Part model, mm, in its own coordinate system. Coordinates: 2 decimals unless noted, no trailing zeros.
from build123d import *

# Parameters (mm, degrees)
SKETCH1_W           = 430
SKETCH1_H           = 500
BOSS_EXTRUDE1_DEPTH = 1.5
SKETCH12_R          = 1.95
CUT_EXTRUDE3_DEPTH  = 50.8
SKETCH6_R           = 1.95
CUT_EXTRUDE4_DEPTH  = 50.8
SKETCH7_R           = 1.95
CUT_EXTRUDE5_DEPTH  = 50.8
FILLET1_R           = 2
CUT_EXTRUDE6_DEPTH  = 10


with BuildPart() as part:
    # Sketch1 → Boss-Extrude1 (new body)
    with BuildSketch(Plane(origin=(0, 0, 0), x_dir=(1, 0, 0), z_dir=(0, 1, 0))):
        Rectangle(SKETCH1_W, SKETCH1_H)
    extrude(amount=BOSS_EXTRUDE1_DEPTH)

    # Sketch12 → Cut-Extrude3 (cut)
    with BuildSketch(Plane(origin=(0, 0, 0), x_dir=(-1, 0, 0), z_dir=(0, -1, 0))):
        with Locations((-185, -175)):
            Circle(SKETCH12_R)
        with Locations((-205, 170)):
            Circle(SKETCH12_R)
        with Locations((-205, -175)):
            Circle(SKETCH12_R)
        with Locations((-185, 170)):
            Circle(SKETCH12_R)
        with Locations((205, -175)):
            Circle(SKETCH12_R)
        with Locations((185, 175)):
            Circle(SKETCH12_R)
        with Locations((205, 175)):
            Circle(SKETCH12_R)
        with Locations((185, -175)):
            Circle(SKETCH12_R)
    extrude(amount=-CUT_EXTRUDE3_DEPTH, mode=Mode.SUBTRACT)

    # Sketch6 → Cut-Extrude4 (cut)
    with BuildSketch(Plane(origin=(0, 1.5, 0), x_dir=(1, 0, 0), z_dir=(0, 1, 0))):
        with Locations((92.292697989, -28)):
            Circle(SKETCH6_R)
        with Locations((42.292697989, -28)):
            Circle(SKETCH6_R)
        with Locations((92.292697989, -178)):
            Circle(SKETCH6_R)
        with Locations((42.292697989, -178)):
            Circle(SKETCH6_R)
    extrude(amount=-CUT_EXTRUDE4_DEPTH, mode=Mode.SUBTRACT)

    # Sketch7 → Cut-Extrude5 (cut)
    with BuildSketch(Plane(origin=(0, 1.5, 0), x_dir=(1, 0, 0), z_dir=(0, 1, 0))):
        with Locations((-114.979961576, 95.192396061)):
            Circle(SKETCH7_R)
        with Locations((-54.979961576, 95.192396061)):
            Circle(SKETCH7_R)
        with Locations((-54.979961576, 0.192396061)):
            Circle(SKETCH7_R)
        with Locations((-114.979961576, 0.192396061)):
            Circle(SKETCH7_R)
    extrude(amount=-CUT_EXTRUDE5_DEPTH, mode=Mode.SUBTRACT)

    # Fillet1
    fillet1_edges = [part.edges().sort_by_distance(p)[0] for p in [
        (215, 0.75, 250),
        (-215, 0.75, 250),
        (-215, 0.75, -250),
        (215, 0.75, -250),
    ]]
    fillet(fillet1_edges, radius=FILLET1_R)

    # Sketch13 → Cut-Extrude6 (cut)
    with BuildSketch(Plane.XZ):
        with BuildLine():
            ThreePointArc((128.328231895, 194.409545443), (128.328231895, 201.480613255), (121.257164083, 201.480613255))
            Line((121.257164083, 201.480613255), (6.257164083, 86.480613255))
            ThreePointArc((6.257164083, 86.480613255), (6.257164083, 79.409545443), (13.328231895, 79.409545443))
            Line((13.328231895, 79.409545443), (128.328231895, 194.409545443))
        make_face()
        with BuildLine():
            ThreePointArc((114.891555161, 206.259007204), (114.891555161, 214.740992796), (106.409569569, 214.740992796))
            Line((106.409569569, 214.740992796), (5.551705193, 113.883128419))
            ThreePointArc((5.551705193, 113.883128419), (5.551705193, 105.401142828), (14.033690785, 105.401142828))
            Line((14.033690785, 105.401142828), (114.891555161, 206.259007204))
        make_face()
        with BuildLine():
            ThreePointArc((128.328231895, 169.409545443), (128.328231895, 176.480613255), (121.257164083, 176.480613255))
            Line((121.257164083, 176.480613255), (6.257164083, 61.480613255))
            ThreePointArc((6.257164083, 61.480613255), (6.257164083, 54.409545443), (13.328231895, 54.409545443))
            Line((13.328231895, 54.409545443), (128.328231895, 169.409545443))
        make_face()
        with BuildLine():
            ThreePointArc((128.328231895, 144.409545443), (128.328231895, 151.480613255), (121.257164083, 151.480613255))
            Line((121.257164083, 151.480613255), (6.257164083, 36.480613255))
            ThreePointArc((6.257164083, 36.480613255), (6.257164083, 29.409545443), (13.328231895, 29.409545443))
            Line((13.328231895, 29.409545443), (128.328231895, 144.409545443))
        make_face()
        with BuildLine():
            ThreePointArc((7.050771569, 137.384062043), (5.156114678, 129.125444121), (13.4147326, 131.020101013))
            Line((13.4147326, 131.020101013), (89.712651072, 207.318019485))
            ThreePointArc((89.712651072, 207.318019485), (89.712651072, 213.681980515), (83.348690041, 213.681980515))
            Line((83.348690041, 213.681980515), (7.050771569, 137.384062043))
        make_face()
        with BuildLine():
            ThreePointArc((128.328231895, 119.409545443), (128.328231895, 126.480613255), (121.257164083, 126.480613255))
            Line((121.257164083, 126.480613255), (6.257164083, 11.480613255))
            ThreePointArc((6.257164083, 11.480613255), (6.257164083, 4.409545443), (13.328231895, 4.409545443))
            Line((13.328231895, 4.409545443), (128.328231895, 119.409545443))
        make_face()
        with BuildLine():
            ThreePointArc((129.178407924, 95.256425689), (129.178407924, 102.327493501), (122.107340112, 102.327493501))
            Line((122.107340112, 102.327493501), (18.815380517, -0.964466094))
            ThreePointArc((18.815380517, -0.964466094), (18.815380517, -8.035533906), (25.886448329, -8.035533906))
            Line((25.886448329, -8.035533906), (129.178407924, 95.256425689))
        make_face()
        with BuildLine():
            ThreePointArc((64.186096271, 206.964466094), (64.186096271, 214.035533906), (57.115028459, 214.035533906))
            Line((57.115028459, 214.035533906), (6.257164083, 163.17766953))
            ThreePointArc((6.257164083, 163.17766953), (6.257164083, 156.106601718), (13.328231895, 156.106601718))
            Line((13.328231895, 156.106601718), (64.186096271, 206.964466094))
        make_face()
        with BuildLine():
            ThreePointArc((128.328231895, 71.106601718), (128.328231895, 78.17766953), (121.257164083, 78.17766953))
            Line((121.257164083, 78.17766953), (42.115028459, -0.964466094))
            ThreePointArc((42.115028459, -0.964466094), (42.115028459, -8.035533906), (49.186096271, -8.035533906))
            Line((49.186096271, -8.035533906), (128.328231895, 71.106601718))
        make_face()
        with BuildLine():
            ThreePointArc((128.434071453, 42.778300689), (128.450410182, 50.077386347), (121.151324524, 50.093725076))
            Line((121.151324524, 50.093725076), (70.101549086, -0.728014801))
            ThreePointArc((70.101549086, -0.728014801), (70.211536159, -8.378376983), (77.854021235, -8.014288369))
            Line((77.854021235, -8.014288369), (80.943634504, -4.5))
            Line((80.943634504, -4.5), (128.434071453, 42.778300689))
        make_face()
        with BuildLine():
            ThreePointArc((39.186096271, 206.964466094), (39.186090231, 214.035539946), (32.11501638, 214.035521827))
            Line((32.11501638, 214.035521827), (28.579518712, 210.5))
            Line((28.579518712, 210.5), (6.257188241, 188.17766953))
            ThreePointArc((6.257188241, 188.17766953), (6.257176162, 181.106613797), (13.328231895, 181.106601718))
            Line((13.328231895, 181.106601718), (39.186096271, 206.964466094))
        make_face()
        with BuildLine():
            ThreePointArc((128.328231895, 21.106601718), (128.328231895, 28.17766953), (121.257164083, 28.17766953))
            Line((121.257164083, 28.17766953), (92.115028459, -0.964466094))
            ThreePointArc((92.115028459, -0.964466094), (92.115028459, -8.035533906), (99.186096271, -8.035533906))
            Line((99.186096271, -8.035533906), (128.328231895, 21.106601718))
        make_face()
        with BuildLine():
            ThreePointArc((128.328449123, -3.893615534), (128.328449135, 3.177669518), (121.257164083, 3.17766953))
            Line((121.257164083, 3.17766953), (117.115028459, -0.964466094))
            ThreePointArc((117.115028459, -0.964466094), (117.11493575, -8.035441194), (124.185910844, -8.035719323))
            Line((124.185910844, -8.035719323), (128.328449123, -3.893615534))
        make_face()
        with BuildLine():
            Line((-60.282225947, -95.192396061), (-54.979961576, -89.89013169))
            Line((-54.979961576, -89.89013169), (-52.328312545, -87.235758493))
            ThreePointArc((-52.328312545, -87.235758493), (-52.33035331, -81.93586188), (-57.630250273, -81.936542135))
            Line((-57.630250273, -81.936542135), (-68.235815502, -92.542107364))
            ThreePointArc((-68.235815502, -92.542107364), (-68.236495757, -97.842004327), (-62.936599144, -97.844045092))
            Line((-62.936599144, -97.844045092), (-60.282225947, -95.192396061))
        make_face()
        with BuildLine():
            Line((-79.432380406, -95.192396061), (-52.328311176, -68.084345475))
            ThreePointArc((-52.328311176, -68.084345475), (-52.332091228, -62.778048343), (-57.638379198, -62.788609103))
            Line((-57.638379198, -62.788609103), (-87.242774375, -92.549084557))
            ThreePointArc((-87.242774375, -92.549084557), (-87.193524879, -97.884311066), (-81.85941362, -97.764626075))
            Line((-81.85941362, -97.764626075), (-79.432380406, -95.192396061))
        make_face()
        with BuildLine():
            Line((-98.589718565, -95.192396061), (-54.979961576, -51.582639071))
            Line((-54.979961576, -51.582639071), (-52.328311176, -48.930599166))
            ThreePointArc((-52.328311176, -48.930599166), (-52.332818712, -43.623576712), (-57.639827781, -43.636319812))
            Line((-57.639827781, -43.636319812), (-106.244222321, -92.550540935))
            ThreePointArc((-106.244222321, -92.550540935), (-106.146641992, -97.928953998), (-100.773557317, -97.670477564))
            Line((-100.773557317, -97.670477564), (-98.589718565, -95.192396061))
        make_face()
        with BuildLine():
            Line((-111.925519092, -89.374450278), (-52.328311147, -29.777242332))
            ThreePointArc((-52.328311147, -29.777242332), (-52.310450744, -24.491922995), (-57.595528665, -24.438342602))
            Line((-57.595528665, -24.438342602), (-117.992839573, -83.224558883))
            ThreePointArc((-117.992839573, -83.224558883), (-118.054977502, -89.353737319), (-111.925519092, -89.374450278))
        make_face()
        with BuildLine():
            Line((-112.328311147, -70.623496023), (-52.374195212, -10.669380088))
            ThreePointArc((-52.374195212, -10.669380088), (-52.374195212, -5.457847361), (-57.58572794, -5.457847361))
            Line((-57.58572794, -5.457847361), (-114.979961576, -62.668544735))
            Line((-114.979961576, -62.668544735), (-117.631612006, -65.320195164))
            ThreePointArc((-117.631612006, -65.320195164), (-117.631612006, -70.623496023), (-112.328311147, -70.623496023))
        make_face()
        with BuildLine():
            Line((-112.328311147, -51.123496023), (-63.949411742, -2.744596618))
            ThreePointArc((-63.949411742, -2.744596618), (-63.936748679, 2.34707829), (-69.028297614, 2.385067165))
            Line((-69.028297614, 2.385067165), (-71.657559216, -0.192396061))
            Line((-71.657559216, -0.192396061), (-114.979961576, -43.514798421))
            Line((-114.979961576, -43.514798421), (-117.432443337, -45.634975273))
            ThreePointArc((-117.432443337, -45.634975273), (-117.726028226, -51.025591461), (-112.328311147, -51.123496023))
        make_face()
        with BuildLine():
            Line((-112.328311147, -31.623496023), (-83.202607923, -2.497792799))
            ThreePointArc((-83.202607923, -2.497792799), (-83.175365618, 2.085432584), (-87.75794332, 2.167155652))
            Line((-87.75794332, 2.167155652), (-117.567824527, -26.25790651))
            ThreePointArc((-117.567824527, -26.25790651), (-117.662945906, -31.591787403), (-112.328311147, -31.623496023))
        make_face()
        with BuildLine():
            Line((-112.328311147, -12.123496023), (-103.048861614, -2.84404649))
            ThreePointArc((-103.048861614, -2.84404649), (-103.048861614, 2.459254369), (-108.352162473, 2.459254369))
            Line((-108.352162473, 2.459254369), (-117.631612006, -6.820195164))
            ThreePointArc((-117.631612006, -6.820195164), (-117.631612006, -12.123496023), (-112.328311147, -12.123496023))
        make_face()
    extrude(amount=-CUT_EXTRUDE6_DEPTH, mode=Mode.SUBTRACT)


solid = part.part
Q1. Cut at A-A on y = 0.6. Count the separate pieces of the cut face and the enclosed holes in it, and give its area (3 significant figures).
Results list:
separate pieces: 1
enclosed holes: 37
area: 196,000 mm2
Q2. Mould opens along Z. For faces 1 (the face through (95.984, 0.74, 25.039)), 2 (the face through (-3, 0, -4)) say: pulls with the +Z half, pulls with the -Z half, needs draft (parallel to the pull), parting line crosses it, or undercut.
Results list:
face 1: undercut
face 2: needs draft
Q3. Wall check: line 1 along Z through (x, y) = (-185, 1.1); line 2 along X through (y, z) = (0.8, 98); line 3 along X through (y, z) = (1.35, -83). Give the ranges that are in metal, low to high.
Results list:
line 1: z = -250 to -176.95, -173.05 to 173.05, 176.95 to 250
line 2: x = -215 to 17.78, 31.92 to 42.78, 56.92 to 67.78, 81.92 to 92.78, 106.92 to 117.78, 130.58 to 215
line 3: x = -215 to -117.76, -105.55 to -96.75, -86.4 to -77.74, -67.24 to -58.69, -51.58 to 215
